For this review, take the finished solid that the model builds, in its own axes (mm). Coordinates: 2 decimals unless noted, no trailing zeros. Loops run counter-clockwise (first coordinate to the right, second up) from the corner with the lowest first, then second, coordinate; pieces in that order, holes last. Notation, with made-up numbers: M -3.5,-13 L 19.5,-13 A7 cw 19.5,0 Z; hole C 78,45 d7. An arc over 180 degrees is marked long. Put each result on its own line as item: value.
Autodesk Inventor part; units mm, degrees
ref_plane "YZ Plane" through (0, 0, 0) normal (1, 0, 0) x (0, 1, 0)
ref_plane "XZ Plane" through (0, 0, 0) normal (0, 1, 0) x (-1, 0, 0)
ref_plane "XY Plane" through (0, 0, 0) normal (0, 0, 1) x (1, 0, 0)
sketch "Sketch1" plane through (0, 0, 0) normal (1, 0, 0) x (0, 1, 0)
  line L0 (12.5, 150) -> (12.5, -150)
  line L1 (12.5, -150) -> (-12.5, -150)
  line L2 (-12.5, -150) -> (-12.5, 150)
  line L3 (-12.5, 150) -> (12.5, 150)
  circle A0 centre (0, 137.5) radius 6
  circle A1 centre (0, -137.5) radius 6
  point P0 (0, 0)
  point P1 (-12.5, 56.5)
  point P2 (-12.5, 60.4432)
  dimension "d0" = 300
  dimension "d1" = 25
  dimension "d2" = 12.5
  dimension "d3" = 150
  dimension "d4" = 12
  dimension "d5" = 12.5
  dimension "d6" = 12
  dimension "d7" = 12.5
extrude "Extrusion1" add sketch "Sketch1" along normal blind 8
full round fillet "Full Round Fillet1" first side at (2.6667, 12.5, -50) centre faces at (2.6667, 4.1667, 150) second side at (2.6667, -12.5, 50)
full round fillet "Full Round Fillet2" first side at (5.3333, 12.5, -54.1666) centre faces at (2.6667, -4.1667, -150) second side at (5.3333, -12.5, 41.6667)
properties part number "Braço Macaco" material "Steel AISI 4142 380 QT"
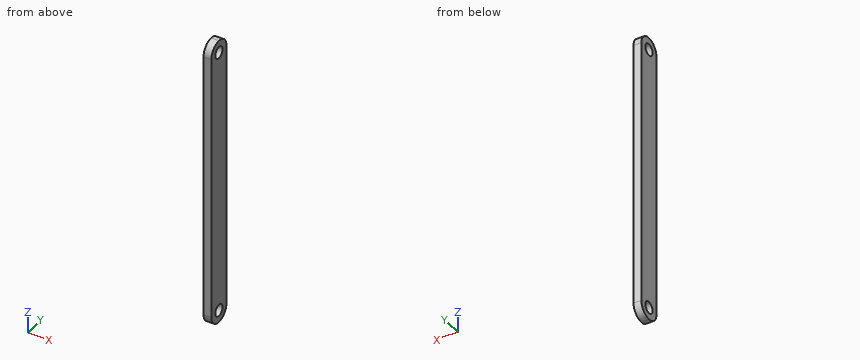
(1) For pin 1 (11 mm diameter, centred on y = 0, z = 137.5, fed in from +X) (3 decimals), flat-tipped, find the tip position at first contact; note if it passes through.
Determined:
pin 1: passes through
(2) Add section B-B (y = 3). Write out the cut boundary in (x, z), plus the area to 3 significant figures.
Determined:
outline: M 0,-149.63 L 8,-149.63 L 8,-142.7 L 0,-142.7 Z; M 0,-132.3 L 8,-132.3 L 8,132.3 L 0,132.3 Z; M 0,142.7 L 8,142.7 L 8,149.63 L 0,149.63 Z
area: 2,230 mm^2
(3) Wall thickness on line 1 along Z through (x, y) = (6, 0); line 2 along Y through (x, z) = (1.25, -137); line 3 along Z through (x, y) = (4.25, 1): over which ranges is each line inside the solid? List them lowest first. Write a range as [from, to].
Determined:
line 1: z = [-150, -143.5], [-131.5, 131.5], [143.5, 150]
line 2: y = [-12.5, -5.98], [5.98, 12.5]
line 3: z = [-149.96, -143.42], [-131.58, 131.58], [143.42, 149.96]
(4) Add section A-A (x = 6.5). State how many separate pieces and enclosed holes the cut face has, plus the area to 3 significant figures.
Determined:
separate pieces: 1
enclosed holes: 2
area: 7,140 mm^2
